The model under review builds one solid part; all positions refer to its coordinate system, in mm. A direction names the side the tool comes from. Give positions to 0.01 mm unless a question says otherwise; leave off trailing zeros. Order: outer loops, then holes, each group sorted by start corner. A loop starts at its lowest first (then second) coordinate and runs counter-clockwise, first axis right, second up.
```python
from build123d import *

# Parameters (mm, degrees)
SKETCH_1_W      = 30
SKETCH_1_H      = 6
SKETCH_1_R      = 2
EXTRUDE_1_DEPTH = 10


with BuildPart() as part:
    # Sketch 1 → Extrude 1 (new body)
    with BuildSketch(Plane(origin=(0, 0, 0), x_dir=(1, 0, 0), z_dir=(0, 1, 0))):
        Polygon((-107.5, 25), (-107.5, -25), (-107.5, -27), (-77.5, -27), (-77.5, -33), (-107.5, -33), (-107.5, -35), (107.5, -35), (107.5, -33), (72.5, -33), (72.5, -27), (107.5, -27), (107.5, -25), (107.5, 25), (72.5, 25), (72.5, 17), (-77.5, 17), (-77.5, 25), align=None)
        with Locations((-32.5, -30)):
            Rectangle(SKETCH_1_W, SKETCH_1_H, mode=Mode.SUBTRACT)
        with Locations((27.5, -30)):
            Rectangle(SKETCH_1_W, SKETCH_1_H, mode=Mode.SUBTRACT)
        with Locations(Location((-75, 12.5, 0), (0, 0, 270))):
            Circle(SKETCH_1_R, mode=Mode.SUBTRACT)
        with Locations(Location((75, 12.5, 0), (0, 0, 270))):
            Circle(SKETCH_1_R, mode=Mode.SUBTRACT)
    extrude(amount=EXTRUDE_1_DEPTH)


solid = part.part
```
Item 1: Clearance check with flat-ended pins moving along their axes: pin 1 Ø3 at (y, z) = (7, 30.5) entering from -X; pin 2 Ø5 at (x, y) = (-55, 4.5) entering from -Z. State where each tip first meets the part, or that it passes through.
Values found:
pin 1: stops at x = -77.5
pin 2: stops at z = -17
Item 2: Take a section at C-C (y = 1.5). Give the boundary of the cut face in (x, z), and give its area (3 significant figures).
Values found:
outline: (-107.5, -25) - (-77.5, -25) - (-77.5, -17) - (72.5, -17) - (72.5, -25) - (107.5, -25) - (107.5, 27) - (72.5, 27) - (72.5, 33) - (107.5, 33) - (107.5, 35) - (-107.5, 35) - (-107.5, 33) - (-77.5, 33) - (-77.5, 27) - (-107.5, 27) - close; hole circle Ø4 at (-75, -12.5); hole (-47.5, 27) - (-17.5, 27) - (-17.5, 33) - (-47.5, 33) - close; hole (12.5, 27) - (42.5, 27) - (42.5, 33) - (12.5, 33) - close; hole circle Ø4 at (75, -12.5)
area: 10,900 mm2
Item 3: For faces 1 (the flat face through (72.5, 5, -21)), 2 (the flat face through (90, 5, 27)), 3 (the flat face through (12.5, 5, 30)), 4 (the flat face through (-77.5, 5, 30)), list the 3-axis set-ups (+Z, -Z, +X, -X, +Y, -Y) from which the entire face can be reached by the end or side of a thin tool; tool diameter is ignored.
Values found:
face 1: -Z, +Y, -Y
face 2: +X, +Y, -Y
face 3: +Y, -Y
face 4: -X, +Y, -Y
Item 4: Draft analysis for pull direction X (two halves, no side actions). For faces 5 (the flat face through (-33, 5, 33)), 6 (the flat face through (-107.5, 5, 1)), 7 (the flat face through (90, 5, -25)), state which applies: released by +X, released by -X, zero draft, split by the parting line, or undercut.
Values found:
face 5: undercut
face 6: released by -X
face 7: zero draft
Item 5: Take a section at A-A (x = 87). Give the boundary of the cut face in (y, z).
Values found:
outline: (0, -25) - (10, -25) - (10, 27) - (0, 27) - close; (0, 33) - (10, 33) - (10, 35) - (0, 35) - close
Item 6: Take a section at B-B (z = -12.5). Give the boundary of the cut face in (x, y), and give its area (3 significant figures).
Values found:
outline: (-107.5, 0) - (-77, 0) - (-77, 10) - (-107.5, 10) - close; (-73, 0) - (73, 0) - (73, 10) - (-73, 10) - close; (77, 0) - (107.5, 0) - (107.5, 10) - (77, 10) - close
area: 2,070 mm2
Item 7: For line 1 (X direction, y = 3.75, z = -12.5); line 2 (Z direction, x = -24, y = 2.5); line 3 (X direction, y = 4.75, z = -13), list the stretches that pass through material, from the lowest coordinate up.
Values found:
line 1: x = -107.5 to -77, -73 to 73, 77 to 107.5
line 2: z = -17 to 27, 33 to 35
line 3: x = -107.5 to -76.94, -73.06 to 73.06, 76.94 to 107.5
Item 8: Take a section at D-D (x = -75). Give the boundary of the cut face in (y, z), and give its area (3 significant figures).
Values found:
outline: (0, -17) - (10, -17) - (10, -14.5) - (0, -14.5) - close; (0, -10.5) - (10, -10.5) - (10, 35) - (0, 35) - close
area: 480 mm2
